Geometry check sheet. Reference: the model listing, model coordinates, mm. Face numbers are marked on the shaded views. Give positions to 0.01 mm unless a question says otherwise; leave off trailing zeros. Write each loop counter-clockwise with the first axis right and the second up, starting at its lowest first coordinate (ties: lowest second). Pieces come first, ordered by that corner, then holes. Notation, with made-up numbers: (4, 74) -> (22, 74) arc R28 cw to (22, 110) -> close; hole circle Ø6 at (4, 26.5). An arc over 180 degrees is marked (long way). Write item = value, one per line. Start each with the question number.
1. Cross-section at C-C, the plane x = 24. Record the cut outline in (y, z), plus the area to 3 significant figures.
2. Mould release check, pull along X, two halves, no side actions. Record for the marked faces 1 and 2: pulls with the +X half, pulls with the -X half, needs draft (parallel to the pull), parting line crosses it, or undercut.
3. Depth check by flat-ended pin: P1, Ø14.5, axis at x = 57.5, y = -3, coming from the -Z side; P2, Ø10, axis at x = 55, z = 2.5, coming from the +Y side; P3, Ø15, axis at x = 0, y = 0, coming from the +Z side; P4, Ø10, axis at x = 46.5, y = 5, coming from the +Z side. Enter the tip coordinate at first touch or a pass-through.
4. Thickness scan on line 1 along Y through (x, z) = (60, -4.5); line 2 along X through (y, z) = (-5.5, -7); line 3 along Z through (x, y) = (24.5, 2.5). Record the ranges inside material, lowest first.
5. Cross-section at B-B, the plane x = 60. Record the cut outline in (y, z), plus the area to 3 significant figures.
6. Cross-section at A-A, the plane x = 0. Record the cut outline in (y, z), plus the area to 3 significant figures.
```python
from build123d import *

# Parameters (mm, degrees)
F0_R         = 12.5
F0_R_2       = 6
F1_DEPTH     = 2.5
F2_DEPTH     = 7.5
F3_DEPTH     = 10
F4_SIZE      = 1
F5_SIZE      = 1
F6_SIZE      = 1
F7_SIZE      = 1
F8_T4_DEPTH  = 74.5908957588
F8_S5_R      = 20
F8_T6_DEPTH  = 39
F8_S7_R      = 10
F8_T8_DEPTH  = 39
F8_T12_DEPTH = 74.5908957588
F8_S13_R     = 20
F8_T14_DEPTH = 39
F8_S15_R     = 10
F8_T16_DEPTH = 39
F8_T20_DEPTH = 74.5908957588
F8_S21_R     = 20
F8_T22_DEPTH = 39
F8_S23_R     = 10
F8_T24_DEPTH = 39
F8_T28_DEPTH = 74.5908957588
F8_S29_R     = 20
F8_T30_DEPTH = 39
F8_S31_R     = 10
F8_T32_DEPTH = 39
F9_T4_ANGLE  = 67.9417369476
F9_T9_ANGLE  = 67.9417369476
F9_T14_ANGLE = 170.4473240821
F9_T20_ANGLE = 67.9417369476
F9_T25_ANGLE = 67.9417369476
F9_T30_ANGLE = 170.4473240821


# Not quite as in the source:
# - a fillet or chamfer that OpenCascade refuses, or shapes differently, is made with other operations: its cross-section is extruded or revolved along the edge and cut away or added


with BuildPart() as f1:
    # F0 (on Top) → F1 (new body, symmetric)
    with BuildSketch(Plane.XY):
        with BuildLine():
            ThreePointArc((3.3333333333, -19.7202659437), (15.2752523165, -12.9099444874), (20, 0))
            ThreePointArc((20, 0), (15.2752523165, 12.9099444874), (3.3333333333, 19.7202659437))
            ThreePointArc((3.3333333333, 19.7202659437), (-20, 0), (3.3333333333, -19.7202659437))
        make_face()
        Circle(F0_R, mode=Mode.SUBTRACT)
        with BuildLine():
            ThreePointArc((3.3333333333, 19.7202659437), (15.2752523165, 12.9099444874), (20, 0))
            ThreePointArc((20, 0), (15.2752523165, -12.9099444874), (3.3333333333, -19.7202659437))
            Line((3.3333333333, -19.7202659437), (61.6666666667, -9.8601329718))
            ThreePointArc((61.6666666667, -9.8601329718), (50, 0), (61.6666666667, 9.8601329718))
            Line((61.6666666667, 9.8601329718), (3.3333333333, 19.7202659437))
        make_face()
        with BuildLine():
            ThreePointArc((70, 0), (67.6376261583, 6.4549722437), (61.6666666667, 9.8601329718))
            ThreePointArc((61.6666666667, 9.8601329718), (50, 0), (61.6666666667, -9.8601329718))
            ThreePointArc((61.6666666667, -9.8601329718), (67.6376261583, -6.4549722437), (70, 0))
        make_face()
        with Locations((60, 0)):
            Circle(F0_R_2, mode=Mode.SUBTRACT)
    extrude(amount=F1_DEPTH, both=True)

    # F0 (on Top) → F2 (join, symmetric)
    with BuildSketch(Plane.XY):
        with BuildLine():
            ThreePointArc((70, 0), (67.6376261583, 6.4549722437), (61.6666666667, 9.8601329718))
            ThreePointArc((61.6666666667, 9.8601329718), (50, 0), (61.6666666667, -9.8601329718))
            ThreePointArc((61.6666666667, -9.8601329718), (67.6376261583, -6.4549722437), (70, 0))
        make_face()
        with Locations((60, 0)):
            Circle(F0_R_2, mode=Mode.SUBTRACT)
    extrude(amount=F2_DEPTH, both=True)

    # F0 (on Top) → F3 (join, symmetric)
    with BuildSketch(Plane.XY):
        with BuildLine():
            ThreePointArc((3.3333333333, -19.7202659437), (15.2752523165, -12.9099444874), (20, 0))
            ThreePointArc((20, 0), (15.2752523165, 12.9099444874), (3.3333333333, 19.7202659437))
            ThreePointArc((3.3333333333, 19.7202659437), (-20, 0), (3.3333333333, -19.7202659437))
        make_face()
        Circle(F0_R, mode=Mode.SUBTRACT)
    extrude(amount=F3_DEPTH, both=True)

    # F4
    f4_edges = [f1.edges().sort_by_distance(p)[0] for p in [
        (-12.5, 0, 10),
        (54, 0, 7.5),
    ]]
    chamfer(f4_edges, length=F4_SIZE)

    # F5
    f5_edges = [f1.edges().sort_by_distance(p)[0] for p in [
        (-12.5, 0, -10),
        (54, 0, 0),
        (66, 0, -1.25),
        (54, 0, -2.5),
        (66, 0, 1.25),
        (54, 0, 2.5),
        (66, 0, -5),
        (54, 0, -7.5),
    ]]
    chamfer(f5_edges, length=F5_SIZE)

    # F6
    f6_edges = [f1.edges().sort_by_distance(p)[0] for p in [
        (-20, 0, -10),
        (50, 0, -7.5),
    ]]
    chamfer(f6_edges, length=F6_SIZE)

    # F7
    f7_edges = [f1.edges().sort_by_distance(p)[0] for p in [
        (-20, 0, 10),
        (50, 0, 7.5),
    ]]
    chamfer(f7_edges, length=F7_SIZE)

    # F8: chamfer of 1 on 5 edges, made by hand


with BuildPart() as f8_tool2:
    # F8_s3 → F8_t4 (new body)
    with BuildSketch(Plane(origin=(65.9404742002, -11.1459744658, 0), x_dir=(0, 0, 1), z_dir=(-0.9860132972, 0.1666666667, 0))):
        Polygon((2.5, 19), (1.5, 20), (2.5, 20), align=None)
    extrude(amount=F8_T4_DEPTH)

    # F8_s5 → F8_t6 (cut, symmetric)
    with BuildSketch(Plane.XY.offset(2)):
        Circle(F8_S5_R)
    extrude(amount=F8_T6_DEPTH, both=True, mode=Mode.SUBTRACT)

    # F8_s7 → F8_t8 (cut, symmetric)
    with BuildSketch(Plane.XY.offset(2)):
        with Locations((60, 0)):
            Circle(F8_S7_R)
    extrude(amount=F8_T8_DEPTH, both=True, mode=Mode.SUBTRACT)


with BuildPart() as f1_1:
    add(f1.part)

    # F8_t1: cut F8_tool2
    add(f8_tool2.part, mode=Mode.SUBTRACT)


with BuildPart() as f8_tool10:
    # F8_s11 → F8_t12 (new body)
    with BuildSketch(Plane(origin=(-7.6071408668, -1.285841494, 0), x_dir=(0, 0, 1), z_dir=(0.9860132972, 0.1666666667, 0))):
        Polygon((2.5, 19), (1.5, 20), (2.5, 20), align=None)
    extrude(amount=F8_T12_DEPTH)

    # F8_s13 → F8_t14 (cut, symmetric)
    with BuildSketch(Plane.XY.offset(2)):
        Circle(F8_S13_R)
    extrude(amount=F8_T14_DEPTH, both=True, mode=Mode.SUBTRACT)

    # F8_s15 → F8_t16 (cut, symmetric)
    with BuildSketch(Plane.XY.offset(2)):
        with Locations((60, 0)):
            Circle(F8_S15_R)
    extrude(amount=F8_T16_DEPTH, both=True, mode=Mode.SUBTRACT)


with BuildPart() as f1_2:
    add(f1_1.part)

    # F8_t9: cut F8_tool10
    add(f8_tool10.part, mode=Mode.SUBTRACT)


with BuildPart() as f8_tool18:
    # F8_s19 → F8_t20 (new body)
    with BuildSketch(Plane(origin=(-7.6071408668, -1.285841494, 0), x_dir=(0, 0, 1), z_dir=(0.9860132972, 0.1666666667, 0))):
        Polygon((-1.5, 20), (-2.5, 19), (-2.5, 20), align=None)
    extrude(amount=F8_T20_DEPTH)

    # F8_s21 → F8_t22 (cut, symmetric)
    with BuildSketch(Plane.XY.offset(-2)):
        Circle(F8_S21_R)
    extrude(amount=F8_T22_DEPTH, both=True, mode=Mode.SUBTRACT)

    # F8_s23 → F8_t24 (cut, symmetric)
    with BuildSketch(Plane.XY.offset(-2)):
        with Locations((60, 0)):
            Circle(F8_S23_R)
    extrude(amount=F8_T24_DEPTH, both=True, mode=Mode.SUBTRACT)


with BuildPart() as f1_3:
    add(f1_2.part)

    # F8_t17: cut F8_tool18
    add(f8_tool18.part, mode=Mode.SUBTRACT)


with BuildPart() as f8_tool26:
    # F8_s27 → F8_t28 (new body)
    with BuildSketch(Plane(origin=(65.9404742002, -11.1459744658, 0), x_dir=(0, 0, 1), z_dir=(-0.9860132972, 0.1666666667, 0))):
        Polygon((-1.5, 20), (-2.5, 19), (-2.5, 20), align=None)
    extrude(amount=F8_T28_DEPTH)

    # F8_s29 → F8_t30 (cut, symmetric)
    with BuildSketch(Plane.XY.offset(-2)):
        Circle(F8_S29_R)
    extrude(amount=F8_T30_DEPTH, both=True, mode=Mode.SUBTRACT)

    # F8_s31 → F8_t32 (cut, symmetric)
    with BuildSketch(Plane.XY.offset(-2)):
        with Locations((60, 0)):
            Circle(F8_S31_R)
    extrude(amount=F8_T32_DEPTH, both=True, mode=Mode.SUBTRACT)


with BuildPart() as f1_4:
    add(f1_3.part)

    # F8_t25: cut F8_tool26
    add(f8_tool26.part, mode=Mode.SUBTRACT)

    # F8_s33 → F8_t34 (revolve, cut)
    with BuildSketch(Plane.XZ):
        Polygon((66.2928932188, 6.7928932188), (66, 6.0857864376), (66, 6.5), align=None)
    revolve(axis=Axis((60, 0, 6.5), (0, 0, 1)), mode=Mode.SUBTRACT)

    # F9: fillet of radius 2 on 10 edges, made by hand


with BuildPart() as f9_tool2:
    # F9_s3 → F9_t4 (revolve)
    with BuildSketch(Plane.XZ):
        with BuildLine():
            ThreePointArc((20, 4.5), (20.5857864376, 3.0857864376), (22, 2.5))
            Line((22, 2.5), (22, 2.46))
            Line((22, 2.46), (19.96, 2.46))
            Line((19.96, 2.46), (19.96, 4.5))
            Line((19.96, 4.5), (20, 4.5))
        make_face()
    revolve(axis=Axis((0, 0, 2.5), (0, 0, -1)), revolution_arc=F9_T4_ANGLE)

    split(bisect_by=Plane(origin=(1.7916666667, -10.5996429447, 10.75), x_dir=(-0.9860132972, -0.1666666667, 0), z_dir=(-0.1178511302, 0.6972166888, -0.7071067812)), keep=Keep.TOP)


with BuildPart() as f1_5:
    add(f1_4.part)

    # F9_t1: union F9_tool2
    add(f9_tool2.part)


with BuildPart() as f9_tool7:
    # F9_s8 → F9_t9 (revolve)
    with BuildSketch(Plane(origin=(0, 0, 0), x_dir=(0, 0, 1), z_dir=(-0.9268024445, 0.3755492362, 0))):
        with BuildLine():
            ThreePointArc((4.5, 20), (3.0857864376, 20.5857864376), (2.5, 22))
            Line((2.5, 22), (2.46, 22))
            Line((2.46, 22), (2.46, 19.96))
            Line((2.46, 19.96), (4.5, 19.96))
            Line((4.5, 19.96), (4.5, 20))
        make_face()
    revolve(axis=Axis((0, 0, 2.5), (0, 0, -1)), revolution_arc=F9_T9_ANGLE)

    split(bisect_by=Plane(origin=(1.7916666667, 10.5996429447, 10.75), x_dir=(0.9860132972, -0.1666666667, 0), z_dir=(-0.1178511302, -0.6972166888, -0.7071067812)), keep=Keep.TOP)


with BuildPart() as f1_6:
    add(f1_5.part)

    # F9_t6: union F9_tool7
    add(f9_tool7.part)


with BuildPart() as f9_tool12:
    # F9_s13 → F9_t14 (revolve)
    with BuildSketch(Plane(origin=(59.5840033564, -4.9786288681, 0), x_dir=(0, 0, 1), z_dir=(0.9965273316, -0.0832663041, 0))):
        with BuildLine():
            ThreePointArc((2.5, 7.0040217561), (3.0857864376, 5.5898081937), (4.5, 5.0040217561))
            Line((4.5, 5.0040217561), (4.5, 4.9640217561))
            Line((4.5, 4.9640217561), (2.46, 4.9640217561))
            Line((2.46, 4.9640217561), (2.46, 7.0040217561))
            Line((2.46, 7.0040217561), (2.5, 7.0040217561))
        make_face()
    revolve(axis=Axis((60, 0, 2.5), (0, 0, -1)), revolution_arc=F9_T14_ANGLE)

    split(bisect_by=Plane(origin=(1.7916666667, 10.5996429447, 10.75), x_dir=(0.9860132972, -0.1666666667, 0), z_dir=(-0.1178511302, -0.6972166888, -0.7071067812)), keep=Keep.TOP)

    split(bisect_by=Plane(origin=(1.7916666667, -10.5996429447, 10.75), x_dir=(-0.9860132972, -0.1666666667, 0), z_dir=(-0.1178511302, 0.6972166888, -0.7071067812)), keep=Keep.TOP)


with BuildPart() as f1_7:
    add(f1_6.part)

    # F9_t11: union F9_tool12
    add(f9_tool12.part)


with BuildPart() as f9_tool18:
    # F9_s19 → F9_t20 (revolve)
    with BuildSketch(Plane(origin=(0, 0, 0), x_dir=(0, 0, 1), z_dir=(-0.9268024445, -0.3755492362, 0))):
        with BuildLine():
            ThreePointArc((-2.5, -22), (-3.0857864376, -20.5857864376), (-4.5, -20))
            Line((-4.5, -20), (-4.5, -19.96))
            Line((-4.5, -19.96), (-2.46, -19.96))
            Line((-2.46, -19.96), (-2.46, -22))
            Line((-2.46, -22), (-2.5, -22))
        make_face()
    revolve(axis=Axis((0, 0, -2.5), (0, 0, 1)), revolution_arc=F9_T20_ANGLE)

    split(bisect_by=Plane(origin=(1.7916666667, -10.5996429447, -10.75), x_dir=(-0.9860132972, -0.1666666667, 0), z_dir=(-0.1178511302, 0.6972166888, 0.7071067812)), keep=Keep.TOP)


with BuildPart() as f1_8:
    add(f1_7.part)

    # F9_t17: union F9_tool18
    add(f9_tool18.part)


with BuildPart() as f9_tool23:
    # F9_s24 → F9_t25 (revolve)
    with BuildSketch(Plane.XZ):
        with BuildLine():
            ThreePointArc((22, -2.5), (20.5857864376, -3.0857864376), (20, -4.5))
            Line((20, -4.5), (19.96, -4.5))
            Line((19.96, -4.5), (19.96, -2.46))
            Line((19.96, -2.46), (22, -2.46))
            Line((22, -2.46), (22, -2.5))
        make_face()
    revolve(axis=Axis((0, 0, -2.5), (0, 0, 1)), revolution_arc=F9_T25_ANGLE)

    split(bisect_by=Plane(origin=(1.7916666667, 10.5996429447, -10.75), x_dir=(0.9860132972, -0.1666666667, 0), z_dir=(-0.1178511302, -0.6972166888, 0.7071067812)), keep=Keep.TOP)


with BuildPart() as f1_9:
    add(f1_8.part)

    # F9_t22: union F9_tool23
    add(f9_tool23.part)


with BuildPart() as f9_tool28:
    # F9_s29 → F9_t30 (revolve)
    with BuildSketch(Plane(origin=(59.5840033564, 4.9786288681, 0), x_dir=(0, 0, 1), z_dir=(0.9965273316, 0.0832663041, 0))):
        with BuildLine():
            ThreePointArc((-2.5, -7.0040217561), (-3.0857864376, -5.5898081937), (-4.5, -5.0040217561))
            Line((-4.5, -5.0040217561), (-4.5, -4.9640217561))
            Line((-4.5, -4.9640217561), (-2.46, -4.9640217561))
            Line((-2.46, -4.9640217561), (-2.46, -7.0040217561))
            Line((-2.46, -7.0040217561), (-2.5, -7.0040217561))
        make_face()
    revolve(axis=Axis((60, 0, -2.5), (0, 0, 1)), revolution_arc=F9_T30_ANGLE)

    split(bisect_by=Plane(origin=(1.7916666667, -10.5996429447, -10.75), x_dir=(-0.9860132972, -0.1666666667, 0), z_dir=(-0.1178511302, 0.6972166888, 0.7071067812)), keep=Keep.TOP)

    split(bisect_by=Plane(origin=(1.7916666667, 10.5996429447, -10.75), x_dir=(0.9860132972, -0.1666666667, 0), z_dir=(-0.1178511302, -0.6972166888, 0.7071067812)), keep=Keep.TOP)


with BuildPart() as f1_10:
    add(f1_9.part)

    # F9_t27: union F9_tool28
    add(f9_tool28.part)


solid = f1_10.part
```
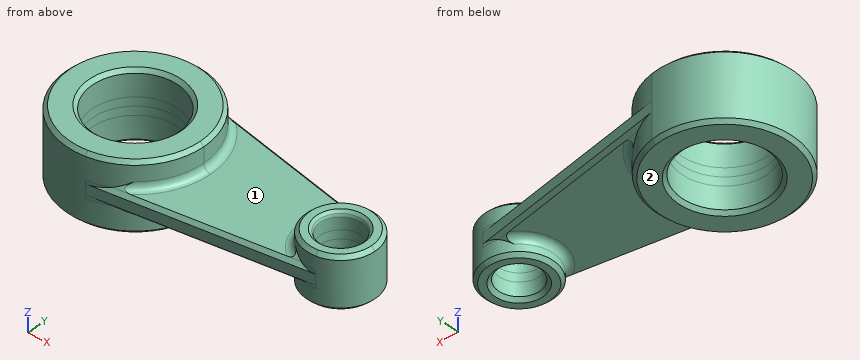
Answers:
q1.outline = (-16.23, -1.5) -> (-15.21, -2.5) -> (15.21, -2.5) -> (16.23, -1.5) -> (16.23, 1.5) -> (15.21, 2.5) -> (-15.21, 2.5) -> (-16.23, 1.5) -> close
q1.area = 160 mm^2
q2.face_1 = undercut
q2.face_2 = needs draft
q3.P1 = -7.5
q3.P2 = 11.82
q3.P3 = through
q3.P4 = 7.1
q4.line_1 = -10 to -6, 6 to 10
q4.line_2 = -19.23 to -11.22, 11.22 to 19.23, 52.25 to 56.54, 63.46 to 67.75
q4.line_3 = -2.5 to 2.5
q5.outline = (-10.14, -1.5) -> (-10, -1.64) -> (-10, -6.5) -> (-9, -7.5) -> (-7, -7.5) -> (-6, -6.5) -> (-6, 6.09) -> (-6.29, 6.79) -> (-7, 7.5) -> (-9, 7.5) -> (-10, 6.5) -> (-10, 1.64) -> (-10.14, 1.5) -> close; (6, -6.5) -> (7, -7.5) -> (9, -7.5) -> (10, -6.5) -> (10, -1.64) -> (10.14, -1.5) -> (10.14, 1.5) -> (10, 1.64) -> (10, 6.5) -> (9, 7.5) -> (7, 7.5) -> (6.29, 6.79) -> (6, 6.09) -> close
q5.area = 117 mm^2
q6.outline = (-20, -9) -> (-19, -10) -> (-13.5, -10) -> (-12.5, -9) -> (-12.5, 9) -> (-13.5, 10) -> (-19, 10) -> (-20, 9) -> close; (12.5, -9) -> (13.5, -10) -> (19, -10) -> (20, -9) -> (20, 9) -> (19, 10) -> (13.5, 10) -> (12.5, 9) -> close
q6.area = 296 mm^2
